from build123d import *

# Parameters (mm, degrees)
F0_R     = 4.445
F1_DEPTH = 9.525
F2_R     = 4.445
F3_DEPTH = 9.525
F4_R     = 4.445
F5_DEPTH = 9.525


with BuildPart() as f1:
    # F0 (on Front) → F1 (new body, symmetric)
    with BuildSketch(Plane.XZ):
        Circle(F0_R)
    extrude(amount=F1_DEPTH, both=True)

    # F2 (on Right) → F3 (join, symmetric)
    with BuildSketch(Plane.YZ):
        Circle(F2_R)
    extrude(amount=F3_DEPTH, both=True)

    # F4 (on Top) → F5 (join, symmetric)
    with BuildSketch(Plane.XY):
        Circle(F4_R)
    extrude(amount=F5_DEPTH, both=True)


solid = f1.part
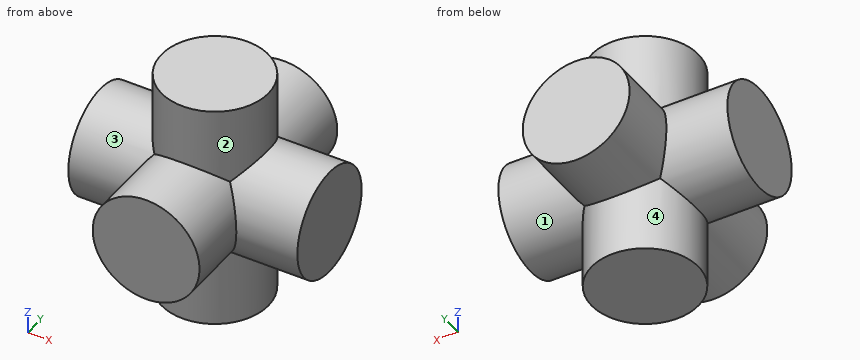
Input: part model. Units: mm. Frame: model coordinates. Face numbers are marked on the shaded views. A direction names the side the tool comes from. Round coordinates to 2 decimals unless told otherwise and drop trailing zeros. Loops run counter-clockwise (first coordinate to the right, second up) from the corner with the lowest first, then second, coordinate; pieces in that order, holes last. Notation, with made-up numbers: M 34.25,83.25 L 68.25,83.25 A22 ccw 68.25,102.25 Z; hole C 44,89 d9. An arc over 180 degrees is marked long. Answer as CSV lines item,"result". Start each with the question number.
(1) Section D-D, the plane x = -4. Output: boundary loops of the cut face in (y, z) (3 decimals), plus the area to 3 significant figures.
(2) Section A-A, the plane x = 0. Output: boundary loops of the cut face in (y, z) (3 decimals), plus the area to 3 significant figures.
(3) Section C-C, the plane z = 7.75. Output: boundary loops of the cut face in (x, y) (3 decimals), plus the area to 3 significant figures.
(4) Reachability of the marked faces 1, 2, 3 and 4 from +Z, -Z, +X, -X, +Y, -Y: full face, straight path, thin tool, end or side. Return the list, or none.
(5) Line query: line 1 (Y direction, x = -6, z = -0.25); line 2 (Y direction, x = -5.5, z = -1.25); line 3 (Z direction, x = 3.25, y = 8.5). Output: solid intervals per line, ascending. Write a range as [from, to].
(6) First-contact query: pin 1 (4 mm diameter, centred on x = -5.5, z = -6, fed in from +Y); pin 2 (1.5 mm diameter, centred on x = -7.5, y = 5.5, fed in from +Z); pin 3 (6 mm diameter, centred on x = -4, y = -6.5, fed in from -Z); pin 4 (5 mm diameter, centred on x = -7, z = -1.5, fed in from -Y) (3 decimals). Flat tips, straight axial feed; report the tip coordinate or a pass-through.
Values found:
1,outline,"M -9.525,-1.939 L -4,-1.939 A4.445 ccw -1.939,-4 L -1.939,-9.525 L 1.939,-9.525 L 1.939,-4 A4.445 ccw 4,-1.939 L 9.525,-1.939 L 9.525,1.939 L 4,1.939 A4.445 ccw 1.939,4 L 1.939,9.525 L -1.939,9.525 L -1.939,4 A4.445 ccw -4,1.939 L -9.525,1.939 Z"
1,area,"143 mm²"
2,outline,"M -9.525,-4.445 L -4.445,-4.445 L -4.445,-9.525 L 4.445,-9.525 L 4.445,-4.445 L 9.525,-4.445 L 9.525,4.445 L 4.445,4.445 L 4.445,9.525 L -4.445,9.525 L -4.445,4.445 L -9.525,4.445 Z"
2,area,"260 mm²"
3,outline,"C 0,0 d8.89"
3,area,"62.1 mm²"
4,face 1,"+X"
4,face 2,"+Z"
4,face 3,"-X"
4,face 4,"-Z"
5,line 1,"y = [-4.44, 4.44]"
5,line 2,"y = [-4.27, 4.27]"
5,line 3,"z = [-3.03, 3.03]"
6,pin 1,"stops at y = 2.74"
6,pin 2,"passes through"
6,pin 3,"stops at z = -4.33"
6,pin 4,"stops at y = -4.445"
